```python
from build123d import *

# Parameters (mm, degrees)
SKETCH1_R               = 7.5
BOSS_EXTRUDE1_DEPTH     = 15
SKETCH2_R               = 7.5
BOSS_EXTRUDE2_DEPTH     = 50
SKETCH3_W               = 50
SKETCH3_H               = 40
BOSS_EXTRUDE3_DEPTH     = 65
CUT_EXTRUDE2_DEPTH      = 96.372952141
SKETCH9_R               = 4
SKETCH9_R_2             = 10.5
CUT_EXTRUDE3_DEPTH      = 104.107953137
CUT_EXTRUDE4_DEPTH      = 92.241437954
CUT_EXTRUDE4_DEPTH_BACK = 92.241437954
SKETCH10_R              = 1.6


with BuildPart() as part:
    # Sketch1 → Boss-Extrude1 (new body)
    with BuildSketch(Plane.XY):
        with BuildLine():
            Line((0, 0), (50, 0))
            Line((50, 0), (50, 50))
            ThreePointArc((50, 50), (40.582575695, 63.228756555), (25, 58.660254038))
            ThreePointArc((25, 58.660254038), (9.417424305, 63.228756555), (0, 50))
            Line((0, 50), (0, 0))
        make_face()
        with Locations((36, 50)):
            Circle(SKETCH1_R, mode=Mode.SUBTRACT)
        with Locations((14, 50)):
            Circle(SKETCH1_R, mode=Mode.SUBTRACT)
    extrude(amount=BOSS_EXTRUDE1_DEPTH)

    # Sketch2 → Boss-Extrude2 (add)
    with BuildSketch(Plane.XY.offset(15)):
        with BuildLine():
            Line((25, 50), (25, 0))
            Line((25, 0), (50, 0))
            Line((50, 0), (50, 50))
            ThreePointArc((50, 50), (37.5, 62.5), (25, 50))
        make_face()
        with Locations((36, 50)):
            Circle(SKETCH2_R, mode=Mode.SUBTRACT)
    extrude(amount=BOSS_EXTRUDE2_DEPTH)

    # Sketch3 → Boss-Extrude3 (add)
    with BuildSketch(Plane(origin=(0, 0, 0), x_dir=(-1, 0, 0), z_dir=(0, 0, -1))):
        with Locations((-25, 20)):
            Rectangle(SKETCH3_W, SKETCH3_H)
    extrude(amount=-BOSS_EXTRUDE3_DEPTH)

    # Sketch2_3 → Cut-Extrude2 (cut, through all)
    with BuildSketch(Plane.XY.offset(15)):
        with BuildLine():
            ThreePointArc((50, 50), (37.5, 62.5), (25, 50))
            ThreePointArc((25, 50), (12.5, 62.5), (0, 50))
            ThreePointArc((0, 50), (9.417424305, 63.228756555), (25, 58.660254038))
            ThreePointArc((25, 58.660254038), (40.582575695, 63.228756555), (50, 50))
        make_face()
    extrude(amount=-CUT_EXTRUDE2_DEPTH, mode=Mode.SUBTRACT)

    # Sketch9 → Cut-Extrude3 (cut, through all)
    with BuildSketch(Plane.ZY):
        with Locations((7, 13)):
            Circle(SKETCH9_R)
        with Locations((58, 13)):
            Circle(SKETCH9_R)
        with Locations((58, 31)):
            Circle(SKETCH9_R)
        with Locations((7, 31)):
            Circle(SKETCH9_R)
        with Locations((32.5, 24)):
            Circle(SKETCH9_R_2)
    extrude(amount=-CUT_EXTRUDE3_DEPTH, mode=Mode.SUBTRACT)

    # Sketch10 → Cut-Extrude4 (cut, two sides: drawn at the far end of the back side and taken through both)
    with BuildSketch(Plane(origin=(0, 40, 0), x_dir=(1, 0, 0), z_dir=(0, 1, 0)).offset(-CUT_EXTRUDE4_DEPTH_BACK)):
        with Locations(Location((9.306144925, -33, 0), (0, 0, 90))):
            Circle(SKETCH10_R)
    extrude(amount=CUT_EXTRUDE4_DEPTH + CUT_EXTRUDE4_DEPTH_BACK, mode=Mode.SUBTRACT)


solid = part.part
```
The model under review builds one solid part; all positions refer to its coordinate system, in mm. A direction names the side the tool comes from. Round coordinates to 2 decimals unless told otherwise and drop trailing zeros. Write each loop counter-clockwise with the first axis right and the second up, starting at its lowest first coordinate (ties: lowest second). Pieces come first, ordered by that corner, then holes. Notation, with made-up numbers: (7, -29.75) - (11, -29.75) arc R14 ccw to (11, -22.75) - close; hole circle Ø4 at (22.5, 69). An arc over 180 degrees is marked (long way). Use one line per item in the form item = value.
Q1. Consider section A-A (z = 58). State the section outline as (x, y) points.
Answer key:
outline = (0, 0) - (50, 0) - (50, 9) - (0, 9) - close; (0, 17) - (50, 17) - (50, 27) - (0, 27) - close; (0, 35) - (50, 35) - (50, 50) arc R12.5 ccw to (25, 50) - (25, 40) - (0, 40) - close; hole circle Ø15 at (36, 50)
Q2. For line 1 (Y direction, x = 17, z = 32.5); line 2 (Y direction, x = 18, z = 58); line 3 (Z direction, x = 37, y = 28), list the stretches that pass through material, from the lowest coordinate up. Write a range as [from, to].
Answer key:
line_1 = [0, 13.5], [34.5, 40]
line_2 = [0, 9], [17, 27], [35, 40]
line_3 = [0, 4.35], [9.65, 22.79], [42.21, 55.35], [60.65, 65]
Q3. Insertion check: pin 1 Ø20 at (x, z) = (17.5, 50.5) entering from +Y; pin 2 Ø8 at (y, z) = (45.5, 46) entering from -X; pin 3 Ø1.5 at (x, z) = (5, 33.5) entering from +Y. Each pin has a flat end and moves straight along its axis. Give the tip position at first contact, or say it passes through.
Answer key:
pin_1 = 57.5
pin_2 = 25
pin_3 = 40
Q4. Consider section D-D (z = 7). State the section outline as (x, y) points.
Answer key:
outline = (0, 0) - (50, 0) - (50, 9) - (0, 9) - close; (0, 17) - (50, 17) - (50, 27) - (0, 27) - close; (0, 35) - (50, 35) - (50, 50) arc R12.5 ccw to (25, 50) arc R12.5 ccw to (0, 50) - close; hole circle Ø15 at (14, 50); hole circle Ø15 at (36, 50)
Q5. Tool access review of faces 5 (the cylindrical face through (10.28, 37.1, 34.27)), 6 (the flat face through (7, 54, 15)): name each direction out of +Z, -Z, +X, -X, +Y, -Y from which nothing blocks a thin tool from reaching the whole face with its end or side.
Answer key:
face_5 = +Y, -Y
face_6 = +Z, -X, +Y
Q6. Draft analysis for pull direction X (two halves, no side actions). For faces 1 (the flat face through (50, 36, 32)), 2 (the cylindrical face through (12.775, 62.497, 7.605)), 3 (the cylindrical face through (24.65, 16.966, 6.479)), 4 (the flat face through (0, 14, 25)), state which applies: +X half, -X half, draft (parallel to the pull), parting line (faces both ways), or undercut.
Answer key:
face_1 = +X half
face_2 = undercut
face_3 = draft
face_4 = -X half
Q7. Consider section B-B (y = 24). State the section outline as (x, z) points, and give its area (3 significant figures).
Answer key:
outline = (0, 0) - (50, 0) - (50, 22) - (0, 22) - close; (0, 43) - (50, 43) - (50, 65) - (0, 65) - close
area = 2,200 mm2
Q8. Consider section C-C (x = 37.5). State the section outline as (y, z) points, and give its area (3 significant figures).
Answer key:
outline = (0, 0) - (42.65, 0) - (42.65, 65) - (0, 65) - close; (57.35, 0) - (62.5, 0) - (62.5, 65) - (57.35, 65) - close; hole circle Ø8 at (13, 7); hole circle Ø8 at (13, 58); hole circle Ø21 at (24, 32.5); hole circle Ø8 at (31, 7); hole circle Ø8 at (31, 58)
area = 2,560 mm2
